```python
from build123d import *

# Parameters (mm, degrees)
ESBO_O1_W                                    = 44
ESBO_O1_H                                    = 38
ESBO_O1_R                                    = 10
RESSALTO_EXTRUS_O1_DEPTH                     = 7
ESBO_O2_R                                    = 15.4
ESBO_O2_R_2                                  = 10
RESSALTO_EXTRUS_O2_DEPTH                     = 2.5
CHANFRO1_SIZE                                = 1
REBAIXO_PARA_PARAFUSO_COM_CABE_A_PAN_2_COUNT = 2
REBAIXO_PARA_PARAFUSO_COM_CABE_A_PAN_2_PITCH = 27
REBAIXO_PARA_PARAFUSO_COM_CABE_A_PAN_3_COUNT = 2
REBAIXO_PARA_PARAFUSO_COM_CABE_A_PAN_3_PITCH = 38.02959374
REBAIXO_PARA_PARAFUSO_COM_CABE_A_PAN_4_COUNT = 2
REBAIXO_PARA_PARAFUSO_COM_CABE_A_PAN_4_PITCH = 24.129857024


with BuildPart() as part:
    # Esboço1 → Ressalto-extrusão1 (new body)
    with BuildSketch(Plane(origin=(0, 0, 0), x_dir=(0, 0, -1), z_dir=(1, 0, 0))):
        with Locations((22, 19)):
            Rectangle(ESBO_O1_W, ESBO_O1_H)
        with Locations((22, 17)):
            Circle(ESBO_O1_R, mode=Mode.SUBTRACT)
    extrude(amount=-RESSALTO_EXTRUS_O1_DEPTH)

    # Esboço2 → Ressalto-extrusão2 (add)
    with BuildSketch(Plane.ZY.offset(7)):
        with Locations((-22, 17)):
            Circle(ESBO_O2_R)
        with Locations(Location((-22, 17, 0), (0, 0, 180))):
            Circle(ESBO_O2_R_2, mode=Mode.SUBTRACT)
    extrude(amount=RESSALTO_EXTRUS_O2_DEPTH)

    # Chanfro1
    chanfro1_edges = [part.edges().sort_by_distance(p)[0] for p in [
        (0, 17, -12),
    ]]
    chamfer(chanfro1_edges, length=CHANFRO1_SIZE)

    # Esboço4 → Rebaixo para parafuso com cabeça panela de M41 (revolve, cut)
    with BuildSketch(Plane(origin=(0, 31, -8.5), x_dir=(0, 0, -1), z_dir=(0, 1, 0))):
        Polygon((0, 0), (0, 9.5), (2.25, 9.5), (2.25, 3.1), (4.5, 3.1), (4.5, 0.025), (4.525, 0), align=None)
    rebaixo_para_parafuso_com_cabe_a_panela = revolve(axis=Axis((6.35, 31, -8.5), (-1, 0, 0)), mode=Mode.SUBTRACT)

    # Rebaixo para parafuso com cabe_a pan 2: Rebaixo para parafuso com cabeça panela de M41 ×2
    with Locations(*[(0, 0, -i * REBAIXO_PARA_PARAFUSO_COM_CABE_A_PAN_2_PITCH) for i in range(1, REBAIXO_PARA_PARAFUSO_COM_CABE_A_PAN_2_COUNT)]):
        add(rebaixo_para_parafuso_com_cabe_a_panela, mode=Mode.SUBTRACT)

    # Rebaixo para parafuso com cabe_a pan 3: Rebaixo para parafuso com cabeça panela de M41 ×2
    with Locations(*[Vector(0, -0.6310874674162201, -0.7757116786991037) * (i * REBAIXO_PARA_PARAFUSO_COM_CABE_A_PAN_3_PITCH) for i in range(1, REBAIXO_PARA_PARAFUSO_COM_CABE_A_PAN_3_COUNT)]):
        add(rebaixo_para_parafuso_com_cabe_a_panela, mode=Mode.SUBTRACT)

    # Rebaixo para parafuso com cabe_a pan 4: Rebaixo para parafuso com cabeça panela de M41 ×2
    with Locations(*[Vector(0, -0.9946184088907778, 0.10360608425945594) * (i * REBAIXO_PARA_PARAFUSO_COM_CABE_A_PAN_4_PITCH) for i in range(1, REBAIXO_PARA_PARAFUSO_COM_CABE_A_PAN_4_COUNT)]):
        add(rebaixo_para_parafuso_com_cabe_a_panela, mode=Mode.SUBTRACT)


solid = part.part
```
Geometry check sheet. Reference: the model listing, model coordinates, mm. A direction names the side the tool comes from. Coordinates: 2 decimals unless noted, no trailing zeros. Loops run counter-clockwise (first coordinate to the right, second up) from the corner with the lowest first, then second, coordinate; pieces in that order, holes last.
Item 1: Sectioned sample at D-D, the plane y = 31. Record the boundary of the cut face in (x, z) (3 decimals).
Item 2: Thickness scan on line 1 (Z direction, x = -0.75, y = 31); line 2 (Z direction, x = -4.55, y = 31); line 3 (Y direction, x = -4.85, z = -38). Record the ranges inside material, lowest first.
Item 3: Sectioned sample at A-A, the plane y = 17. Record the boundary of the cut face in (x, z), then the cut area to 3 significant figures.
Item 4: Sectioned sample at B-B, the plane x = -6. Record the boundary of the cut face in (y, z), then the cut area to 3 significant figures.
Item 5: Sectioned sample at C-C, the plane z = -22. Record the boundary of the cut face in (x, y).
Item 6: Go/stop test with flat-tipped pins: pin 1 Ø5 at (y, z) = (31, -35.5) entering from +X; pin 2 Ø18 at (y, z) = (17, -22) entering from -X; pin 3 Ø6 at (y, z) = (7, -6) entering from -X. Record where each tip stops, or that it passes through.
Item 7: Release check for a two-part mould opening along Y. For faces 1 (the face through (-5.023, 8.369, -4.214)), 2 (the face through (0, 28, -17)), 3 (the face through (-3, 38, -22)), 4 (the face through (-5.023, 32.369, -6.714)) record: released by +Y, released by -Y, zero draft, split by the parting line, or undercut.
Item 8: Access from +Z, -Z, +X, -X, +Y, -Y to the whole of each face (thin tool, end or side, straight path). Record for faces 5 (the face through (-8.232, 1.966, -25.338)), 6 (the face through (-3.1, 32, -38)), 7 (the face through (-9.5, 7, -19)).
Check result:
1. outline: (-9.5, -28.416) - (-7, -28.416) - (-7, -33.25) - (-3.1, -33.25) - (-3.1, -31) - (-0.025, -31) - (0, -30.975) - (0, -13.025) - (-0.025, -13) - (-3.1, -13) - (-3.1, -10.75) - (-7, -10.75) - (-7, -15.584) - (-9.5, -15.584) - close; (-7, -44) - (0, -44) - (0, -40.025) - (-0.025, -40) - (-3.1, -40) - (-3.1, -37.75) - (-7, -37.75) - close; (-7, -6.25) - (-3.1, -6.25) - (-3.1, -4) - (-0.025, -4) - (0, -3.975) - (0, 0) - (-7, 0) - close
2. line 1: z = -44 to -40, -31 to -13, -4 to 0
2. line 2: z = -44 to -37.75, -33.25 to -10.75, -6.25 to 0
2. line 3: y = 0 to 4.75, 9.25 to 38
3. outline: (-9.5, -37.4) - (-7, -37.4) - (-7, -44) - (0, -44) - (0, -33) - (-1, -32) - (-9.5, -32) - close; (-9.5, -12) - (-1, -12) - (0, -11) - (0, 0) - (-7, 0) - (-7, -6.6) - (-9.5, -6.6) - close
3. area: 194 mm2
4. outline: (0, -44) - (38, -44) - (38, 0) - (0, 0) - close; hole circle Ø4.5 at (7, -38); hole circle Ø4.5 at (7, -6); hole circle Ø20 at (17, -22); hole circle Ø4.5 at (31, -35.5); hole circle Ø4.5 at (31, -8.5)
4. area: 1,290 mm2
5. outline: (-9.5, 1.6) - (-7, 1.6) - (-7, 0) - (0, 0) - (0, 6) - (-1, 7) - (-9.5, 7) - close; (-9.5, 27) - (-1, 27) - (0, 28) - (0, 38) - (-7, 38) - (-7, 32.4) - (-9.5, 32.4) - close
6. pin 1: stops at x = -3.1
6. pin 2: passes through
6. pin 3: stops at x = -7
7. face 1: undercut
7. face 2: zero draft
7. face 3: released by +Y
7. face 4: undercut
8. face 5: -X
8. face 6: +X
8. face 7: +Z, -Z, -X, +Y, -Y
